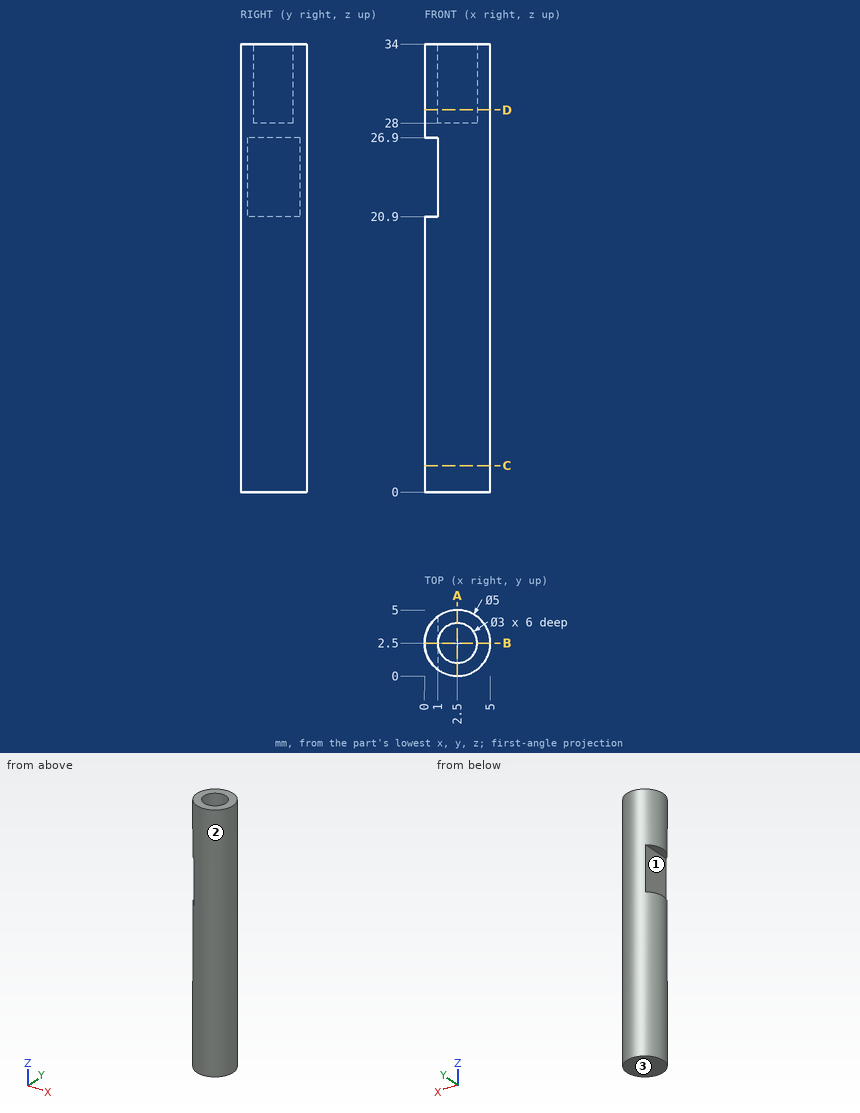
Answer from the drawing. Dimensions are ordinates in mm from the lowest x, y and z of the part. Round coordinates to 2 decimals unless told otherwise and drop trailing zeros. Loops run counter-clockwise (first coordinate to the right, second up) from the corner with the lowest first, then second, coordinate; pieces in that order, holes last.
(1) The part is cut by section B-B, the plane y = 2.5. Give the vertices of the cut face in (x, z).
Computed values:
outline: (0, 0) - (5, 0) - (5, 34) - (4, 34) - (4, 28) - (1, 28) - (1, 34) - (0, 34) - (0, 26.9) - (1, 26.9) - (1, 20.9) - (0, 20.9) - close
(2) Find the intervals of material crossed by L1, parallel to Y at x = 2.5, z = 29.7; L2, parallel to Z at x = 3, y = 3.4; L3, parallel to X at y = 0.5, z = 7, in increasing order.
Computed values:
L1: y = 0 to 1, 4 to 5
L2: z = 0 to 28
L3: x = 1 to 4
(3) The mould has two halves that part along Z. Classify the marked faces 1, 2 and 3: pulls with the +Z half, pulls with the -Z half, needs draft (parallel to the pull), parting line crosses it, or undercut.
Computed values:
face 1: undercut
face 2: needs draft
face 3: pulls with the -Z half
(4) Each of these flat-tipped pins is pushed along its axis until it touches: P1, Ø1, axis at y = 4, z = 20, coming from the -X side; P2, Ø1.5, axis at x = 3.5, z = 29.5, coming from the -Y side; P3, Ø1, axis at x = 4, z = 26.5, coming from the -Y side. Where does it stop, or does it pass through?
Computed values:
P1: stops at x = 0.21
P2: stops at y = 0.01
P3: stops at y = 0.21
(5) The part is cut by section A-A, the plane x = 2.5. Give the vertices of the cut face in (y, z), and give its area (3 significant figures).
Computed values:
outline: (0, 0) - (5, 0) - (5, 34) - (4, 34) - (4, 28) - (1, 28) - (1, 34) - (0, 34) - close
area: 152 mm2
(6) The part is cut by section C-C, the plane z = 2. Give the vertices of the cut face in (x, y).
Computed values:
outline: circle Ø5 at (2.5, 2.5)
(7) The part is cut by section D-D, the plane z = 29. Give the vertices of the cut face in (x, y), and give its area (3 significant figures).
Computed values:
outline: circle Ø5 at (2.5, 2.5); hole circle Ø3 at (2.5, 2.5)
area: 12.6 mm2
